CAD build for the part. Positions are in the model's coordinates, mm. A direction names the side the tool comes from. Give positions to 0.01 mm unless a question says otherwise; leave off trailing zeros. Order: outer loops, then holes, each group sorted by start corner. A loop starts at its lowest first (then second) coordinate and runs counter-clockwise, first axis right, second up. Notation, with made-up numbers: M 34,33.5 L 91,33.5 A34 ccw 91,67.5 Z; hole C 63,-27 d11. An arc over 180 degrees is marked long. Put each result on its own line as item: value. Start each with the question number.
1) Cut at B-B (y = 0). Write the cut outline in (x, z), and give its area (3 significant figures).
2) Cut at C-C (z = 0.85). Write the cut outline in (x, y).
3) Pin check, flat tips, straight feed: pin 1 (1.5 mm diameter, centred on x = -8, y = 54, fed in from +Z); pin 2 (1 mm diameter, centred on x = -72, z = 1, fed in from -Y). Stop position of each tip, or through.
4) Drill centre lines: line 1 (Y direction, x = -2.16, z = 1.5); line 2 (Z direction, x = -30.5, y = 49); line 3 (X direction, y = -5.5, z = 1.2). Where is each one in solid material? Low to high. Write a range as [from, to].
5) Tool access for faces 1 (the face through (49, 1, 2)), 2 (the face through (-60.6, -55.9, 1)): list every direction of +Z, -Z, +X, -X, +Y, -Y with a clear straight run to the whole face (end or side of a thin tool).
6) Cut at A-A (x = -2.16). Write the cut outline in (y, z), and give its area (3 significant figures).
7) Two-plate mould, pull along X, no slides. Class faces 3 (the face through (44.53, 15.02, 2.49)), 4 (the face through (-21.533, 62.743, 1.014)), 5 (the face through (16, 1, 0)): released by +X, released by -X, zero draft, split by the parting line, or undercut.
8) Cut at D-D (x = 35.5). Write the cut outline in (y, z), and give its area (3 significant figures).
```python
from build123d import *

# Parameters (mm, degrees)
F0_W      = 150
F0_H      = 140
F1_DEPTH  = 2
F3_DEPTH  = 2.001
F5_DEPTH  = 2.001
F7_DEPTH  = 2.001
F8_R      = 50
F9_DEPTH  = 1
F10_R     = 12.75
F11_DEPTH = 25


with BuildPart() as f1:
    # F0 (on Top) → F1 (new body)
    with BuildSketch(Plane.XY):
        Rectangle(F0_W, F0_H)
    extrude(amount=F1_DEPTH)

    # F2 (on face) → F3 (cut, through all)
    with BuildSketch(Plane.XY.offset(2)):
        Polygon((-75, 70), (-75, 41.5), (-46.5, 70), align=None)
        Polygon((-46.5, -70), (-75, -41.5), (-75, -70), align=None)
    extrude(amount=-F3_DEPTH, mode=Mode.SUBTRACT)

    # F4 (on face) → F5 (cut, through all)
    with BuildSketch(Plane.XY.offset(2)):
        with BuildLine():
            Line((-69.68, 9.5), (-75, 9.5))
            Line((-75, 9.5), (-75, -9.5))
            Line((-75, -9.5), (-69.68, -9.5))
            ThreePointArc((-69.68, -9.5), (-67.912233, -8.767767), (-67.18, -7))
            Line((-67.18, -7), (-67.18, 7))
            ThreePointArc((-67.18, 7), (-67.912233, 8.767767), (-69.68, 9.5))
        make_face()
    extrude(amount=-F5_DEPTH, mode=Mode.SUBTRACT)

    # F6 (on face) → F7 (cut, through all)
    with BuildSketch(Plane.XY.offset(2)):
        with BuildLine():
            Line((-28.031671, -70), (-15, -70))
            Line((-15, -70), (-16.416769, -66.495551))
            ThreePointArc((-16.416769, -66.495551), (-21.515836, -63.056988), (-26.614902, -66.495551))
            Line((-26.614902, -66.495551), (-28.031671, -70))
        make_face()
        with BuildLine():
            Line((-27.876137, 70), (-26.631231, 66.430881))
            ThreePointArc((-26.631231, 66.430881), (-21.438069, 62.742254), (-16.244907, 66.430881))
            Line((-16.244907, 66.430881), (-15, 70))
            Line((-15, 70), (-27.876137, 70))
        make_face()
    extrude(amount=-F7_DEPTH, mode=Mode.SUBTRACT)

    # F8 (on face) → F9 (join)
    with BuildSketch(Plane.XY.offset(2)):
        with Locations((-3.16, 0)):
            Circle(F8_R)
    extrude(amount=F9_DEPTH)

    # F10 (on face) → F11 (cut)
    with BuildSketch(Plane.XY.offset(3)):
        with Locations((-2.16, 0)):
            Circle(F10_R)
    extrude(amount=-F11_DEPTH, mode=Mode.SUBTRACT)


solid = f1.part
```
Solution:
1. outline: M -67.18,0 L -14.91,0 L -14.91,3 L -53.16,3 L -53.16,2 L -67.18,2 Z; M 10.59,0 L 75,0 L 75,2 L 46.84,2 L 46.84,3 L 10.59,3 Z
1. area: 308 mm²
2. outline: M -75,-41.5 L -46.5,-70 L -28.03,-70 L -26.61,-66.5 A5.5 cw -16.42,-66.5 L -15,-70 L 75,-70 L 75,70 L -15,70 L -16.24,66.43 A5.5 cw -26.63,66.43 L -27.88,70 L -46.5,70 L -75,41.5 L -75,9.5 L -69.68,9.5 A2.5 cw -67.18,7 L -67.18,-7 A2.5 cw -69.68,-9.5 L -75,-9.5 Z; hole C -2.16,0 d25.5
3. pin 1: z = 2
3. pin 2: y = -45
4. line 1: [-70, -12.75], [12.75, 70]
4. line 2: [0, 2]
4. line 3: [-67.18, -13.66], [9.34, 75]
5. face 1: +Z
5. face 2: +Z, -Z, -X, -Y
6. outline: M -70,0 L -12.75,0 L -12.75,3 L -49.99,3 L -49.99,2 L -70,2 Z; M 12.75,0 L 70,0 L 70,2 L 49.99,2 L 49.99,3 L 12.75,3 Z
6. area: 303 mm²
7. face 3: split by the parting line
7. face 4: undercut
7. face 5: zero draft
8. outline: M -70,0 L 70,0 L 70,2 L 31.71,2 L 31.71,3 L -31.71,3 L -31.71,2 L -70,2 Z
8. area: 343 mm²
